Source: CAD feature listing. Evaluate the final solid. Frame: model axes, mm. A direction names the side the tool comes from. Round coordinates to 2 decimals unless told otherwise and drop trailing zeros. Write each loop counter-clockwise with the first axis right and the second up, starting at its lowest first coordinate (ties: lowest second). Pieces come first, ordered by that corner, then holes. Notation, with made-up numbers: (11.25, 4) - (58.25, 4) arc R21 cw to (58.25, 31) - close; hole circle Ø1 at (-0.5, 22.25). An arc over 180 degrees is marked (long way). Write item = value, one per line. Start each with the question number.
```python
from build123d import *

# Parameters (mm, degrees)
SKETCH1_R           = 3
SKETCH1_R_2         = 2.5
BOSS_EXTRUDE1_DEPTH = 20
SKETCH1_3_R         = 5
SKETCH1_3_R_2       = 3
BOSS_EXTRUDE2_DEPTH = 5
SKETCH4_W           = 5
SKETCH4_H           = 5
CUT_EXTRUDE2_DEPTH  = 1
SKETCH5_W           = 5
SKETCH5_H           = 5
CUT_EXTRUDE3_DEPTH  = 1
SKETCH6_W           = 5
SKETCH6_H           = 5
CUT_EXTRUDE4_DEPTH  = 1
SKETCH7_W           = 5
SKETCH7_H           = 5
CUT_EXTRUDE5_DEPTH  = 1


with BuildPart() as part:
    # Sketch1 → Boss-Extrude1 (new body)
    with BuildSketch(Plane(origin=(0, 0, 0), x_dir=(1, 0, 0), z_dir=(0, 1, 0))):
        with Locations(Location((0, 0, 0), (0, 0, 270))):
            Circle(SKETCH1_R)
        with Locations(Location((0, 0, 0), (0, 0, 270))):
            Circle(SKETCH1_R_2, mode=Mode.SUBTRACT)
    extrude(amount=BOSS_EXTRUDE1_DEPTH)

    # Sketch1_3 → Boss-Extrude2 (add)
    with BuildSketch(Plane(origin=(0, 0, 0), x_dir=(1, 0, 0), z_dir=(0, 1, 0))):
        with Locations(Location((0, 0, 0), (0, 0, 270))):
            Circle(SKETCH1_3_R)
        with Locations(Location((0, 0, 0), (0, 0, 270))):
            Circle(SKETCH1_3_R_2, mode=Mode.SUBTRACT)
    extrude(amount=BOSS_EXTRUDE2_DEPTH)

    # Sketch4 → Cut-Extrude2 (cut)
    with BuildSketch(Plane.XY.offset(5)):
        with Locations((0, 2.5)):
            Rectangle(SKETCH4_W, SKETCH4_H)
    extrude(amount=-CUT_EXTRUDE2_DEPTH, mode=Mode.SUBTRACT)

    # Sketch5 → Cut-Extrude3 (cut)
    with BuildSketch(Plane.ZY.offset(5)):
        with Locations((0, 2.5)):
            Rectangle(SKETCH5_W, SKETCH5_H)
    extrude(amount=-CUT_EXTRUDE3_DEPTH, mode=Mode.SUBTRACT)

    # Sketch6 → Cut-Extrude4 (cut)
    with BuildSketch(Plane(origin=(0, 0, -5), x_dir=(-1, 0, 0), z_dir=(0, 0, -1))):
        with Locations((0, 2.5)):
            Rectangle(SKETCH6_W, SKETCH6_H)
    extrude(amount=-CUT_EXTRUDE4_DEPTH, mode=Mode.SUBTRACT)

    # Sketch7 → Cut-Extrude5 (cut)
    with BuildSketch(Plane(origin=(5, 0, 0), x_dir=(0, 0, -1), z_dir=(1, 0, 0))):
        with Locations((0, 2.5)):
            Rectangle(SKETCH7_W, SKETCH7_H)
    extrude(amount=-CUT_EXTRUDE5_DEPTH, mode=Mode.SUBTRACT)


solid = part.part
```
(1) Section D-D (x = 2.75). Return the cut outline in (y, z).
(2) Reachability of faces 5 (the flat face through (0, 3, -4)), 6 (the flat face through (1, 5, -3)), 7 (the flat face through (-4, 3, 0)), 8 (the flat face through (0, 3, 4)) from +Z, -Z, +X, -X, +Y, -Y: full face, straight path, thin tool, end or side. Return the list, or none.
(3) Section C-C (y = 13.75). Return the cut outline in (x, z).
(4) Section B-B (z = -1.75). Return the cut outline in (x, y), plus the area to 3 significant figures.
(5) Contact query for flat-ended pins moving along their axis: P1, Ø2, axis at y = 7, z = -1.5, coming from the +X side; P2, Ø1.5, axis at x = 0, y = 8.5, coming from the +Z side; P3, Ø5, axis at y = 16, z = 1.5, coming from the -X side. Output: stop coordinate, or through.
(6) Section A-A (x = 0). Return the cut outline in (y, z), plus the area to 3 significant figures.
(7) Ray query, L1, parallel to X at y = 9.25, z = 0; L2, parallel to X at y = 4.5, z = 0; L3, parallel to Y at x = 2.5, z = -2. Return the intervals inside material, ascending. Write a range as from..to.
(8) Pull-direction query (X, two-part tool) for faces 1 (the cylindrical face through (3.52, 2.46, 3.55)), 2 (the cylindrical face through (0.9, 12.4, 2.86)), 3 (the cylindrical face through (-2.44, 9.86, -0.54)), 4 (the cylindrical face through (-3.55, 2.46, 3.52)); classes: +X half, -X half, draft (parallel to the pull), parting line (faces both ways), or undercut.
Solution:
q1.outline = (0, -4.18) - (5, -4.18) - (5, -1.2) - (20, -1.2) - (20, 1.2) - (5, 1.2) - (5, 4.18) - (0, 4.18) - close
q2.face_5 = -Z, +Y, -Y
q2.face_6 = +Y
q2.face_7 = -X, +Y, -Y
q2.face_8 = +Z, +Y, -Y
q3.outline = circle Ø6 at (0, 0); hole circle Ø5 at (0, 0)
q4.outline = (-4, 0) - (-1.79, 0) - (-1.79, 20) - (-2.44, 20) - (-2.44, 5) - (-4, 5) - close; (1.79, 0) - (4, 0) - (4, 5) - (2.44, 5) - (2.44, 20) - (1.79, 20) - close
q4.area = 41.7 mm^2
q5.P1 = 2.96
q5.P2 = 3
q5.P3 = -3
q6.outline = (0, -4) - (5, -4) - (5, -3) - (20, -3) - (20, -2.5) - (0, -2.5) - close; (0, 2.5) - (20, 2.5) - (20, 3) - (5, 3) - (5, 4) - (0, 4) - close
q6.area = 30.0 mm^2
q7.L1 = -3..-2.5, 2.5..3
q7.L2 = -4..-2.5, 2.5..4
q7.L3 = 0..5
q8.face_1 = +X half
q8.face_2 = parting line
q8.face_3 = undercut
q8.face_4 = -X half
